Read the model definition and answer for the solid it produces. Units are mm, in the model's axes. A direction names the side the tool comes from. Coordinates: 2 decimals unless noted, no trailing zeros. Order: outer loops, then holes, each group sorted by start corner. A loop starts at its lowest first (then second) coordinate and runs counter-clockwise, first axis right, second up. Notation, with made-up numbers: (7, 26) - (46, 26) arc R12 cw to (46, 36) - close; hole circle Ø1 at (18.5, 30.25). An arc over 180 degrees is marked (long way). Use one line per item in the form item = value.
Autodesk Inventor part; units mm, degrees
ref_plane "YZ Plane" through (0, 0, 0) normal (1, 0, 0) x (0, 1, 0)
ref_plane "XZ Plane" through (0, 0, 0) normal (0, 1, 0) x (-1, 0, 0)
ref_plane "XY Plane" through (0, 0, 0) normal (0, 0, 1) x (1, 0, 0)
sketch "Sketch1" plane through (0, 0, 0) normal (0, 0, 1) x (1, 0, 0)
  line L0 (0, 0) -> (440, 0)
  line L1 (440, 0) -> (440, 75)
  line L2 (440, 75) -> (0, 75)
  line L3 (0, 75) -> (0, 0)
  dimension "d0" = 75
  dimension "d1" = 440
extrude "Extrusion1" add sketch "Sketch1" along normal blind 8
sketch "Sketch2" plane through (0, 0, 8) normal (0, 0, 1) x (1, 0, 0)
  line L0 (0, 0) -> (0, 75)
  line L1 (440, 0) -> (0, 0)
  circle A0 centre (70, 25) radius 14
  line L2 (59, 16.3397) -> (59, 0)
  line L3 (81, 16.3397) -> (81, 0)
  circle A1 centre (220, 25) radius 14
  line L4 (209, 16.3397) -> (209, 0)
  line L5 (231, 16.3397) -> (231, 0)
  circle A2 centre (370, 25) radius 14
  line L6 (359, 16.3397) -> (359, 0)
  line L7 (381, 16.3397) -> (381, 0)
  line L8 (209, 0) -> (231, 0)
  line L9 (359, 0) -> (381, 0)
  line L10 (521.97, 0) -> (544.83, 0)
  line L11 (671.8667, 0) -> (697.23, 0)
  line L12 (826.77, 0) -> (849.63, 0)
  line L13 (674.37, 0) -> (697.23, 0)
  dimension "d4" = 22
  dimension "d5" = 11
  dimension "d7" = 25
  dimension "d8" = 28
  dimension "d9" = 70
  dimension "d17" = 150
  dimension "d58" = 440
extrude "Extrusion4" cut sketch "Sketch2" against normal up to next
sketch "Sketch3" plane through (0, 0, 8) normal (0, 0, 1) x (1, 0, 0)
  arc A0 (81, 16.3397) -> (59, 16.3397) centre (70, 25) ccw
  circle A1 centre (70, 25) radius 19
  line L0 (209, 0) -> (81, 0)
  point P0 (70, 44)
  point P1 (53.5455, 15.5)
  point P2 (86.4545, 15.5)
  point P3 (220, 44)
  point P4 (236.4545, 15.5)
  point P5 (203.5455, 15.5)
  point P6 (370, 44)
  point P7 (386.4545, 15.5)
  point P8 (353.5455, 15.5)
  dimension "d59" = 38
  dimension "d62" = 360
  dimension "d66" = 150
hole "Hole1" at (70, 44, 8) at (86.4545, 15.5, 8) at (53.5455, 15.5, 8) at (203.5455, 15.5, 8) at (236.4545, 15.5, 8) at (220, 44, 8) at (353.5455, 15.5, 8) at (370, 44, 8) at (386.4545, 15.5, 8) direction (0, 0, -1) diameter 7.7978 end through all
sketch "Sketch4" plane through (0, 0, 8) normal (0, 0, 1) x (1, 0, 0)
  line L0 (440, 75) -> (440, 0)
  line L1 (0, 0) -> (0, 75)
  line L2 (440, 0) -> (0, 0)
  point P0 (59, 0)
  point P1 (5, 69)
  point P2 (5, 6)
  point P3 (435, 6)
  point P4 (435, 69)
  dimension "d42" = 6
  dimension "d44" = 5
  dimension "d45" = 5
  dimension "d71" = 69
hole "Hole2" at (5, 69, 8) at (5, 6, 8) at (435, 6, 8) at (435, 69, 8) direction (0, 0, -1) diameter 4.5 end through all counterbore diameter 8 counterbore depth 4
equation "\"d4\" = 2 * d5"
equation "\"d9\" = -d17 + 0.5 * d58"
properties part number "Top" material "Aluminum-6061"
(1) Section C-C, the plane y = 44 is taken. Write down the section's boundary in (x, z), then the cut area to 3 significant figures.
Answer list:
outline = (0, 0) - (66.1, 0) - (66.1, 8) - (0, 8) - close; (73.9, 0) - (216.1, 0) - (216.1, 8) - (73.9, 8) - close; (223.9, 0) - (366.1, 0) - (366.1, 8) - (223.9, 8) - close; (373.9, 0) - (440, 0) - (440, 8) - (373.9, 8) - close
area = 3,330 mm2
(2) Section D-D, the plane z = 6.75 is taken. State how many separate pieces and enclosed holes the cut face has, then the cut area to 3 significant figures.
Answer list:
separate_pieces = 1
enclosed_holes = 13
area = 29,700 mm2
(3) Section A-A, the plane y = 25 is taken. Write down the section's boundary in (x, z), then the cut area to 3 significant figures.
Answer list:
outline = (0, 0) - (56, 0) - (56, 8) - (0, 8) - close; (84, 0) - (206, 0) - (206, 8) - (84, 8) - close; (234, 0) - (356, 0) - (356, 8) - (234, 8) - close; (384, 0) - (440, 0) - (440, 8) - (384, 8) - close
area = 2,850 mm2
(4) Section B-B, the plane x = 70 is taken. Write down the section's boundary in (y, z).
Answer list:
outline = (39, 0) - (40.1, 0) - (40.1, 8) - (39, 8) - close; (47.9, 0) - (75, 0) - (75, 8) - (47.9, 8) - close
(5) Which of the six approach directions +Z, -Z, +X, -X, +Y, -Y give full straight-line access (tool end or side, diameter ignored) to faces 4 (the cylindrical face through (57.35, 16.35, 3.94)), 5 (the cylindrical face through (6.532, 65.305, 5.972)), 6 (the flat face through (59, 8, 4))?
Answer list:
face_4 = +Z, -Z
face_5 = +Z
face_6 = +Z, -Z, -Y
(6) Straight lines are drawn through the part: L1, parallel to Y at x = 435, z = 5.95; L2, parallel to X at y = 44, z = 4; L3, parallel to X at y = 24.5, z = 4.5. For each, find the intervals that lie inside material, in ascending order.
Answer list:
L1 = 0 to 2, 10 to 65, 73 to 75
L2 = 0 to 66.1, 73.9 to 216.1, 223.9 to 366.1, 373.9 to 440
L3 = 0 to 56.01, 83.99 to 206.01, 233.99 to 356.01, 383.99 to 440
(7) Given pin 1 Ø5 at (x, y) = (5, 6) entering from +Z, flat-ended and moving along its own axis, determine where the tip first touches the part or whether it passes through.
Answer list:
pin_1 = 4
(8) The mould has two halves that part along X. Classify faces 1 (the flat face through (231, 8, 4)), 2 (the flat face through (223, 75, 4)), 3 (the flat face through (440, 37, 4)): +X half, -X half, draft (parallel to the pull), parting line (faces both ways), or undercut.
Answer list:
face_1 = undercut
face_2 = draft
face_3 = +X half
